```python
from build123d import *

# Parameters (mm, degrees)
F1_DEPTH = 11
F3_DEPTH = 4
F5_D     = 5


with BuildPart() as f1:
    # F0 (on Top) → F1 (new body)
    with BuildSketch(Plane.XY):
        with BuildLine():
            Line((-1.5, 17.95), (-1.5, 14.874559))
            ThreePointArc((-1.5, 14.874559), (0, -14.95), (1.5, 14.874559))
            Line((1.5, 14.874559), (1.5, 17.95))
            Line((1.5, 17.95), (-1.5, 17.95))
        make_face()
    extrude(amount=F1_DEPTH)

    # F2 (on face) → F3 (join)
    with BuildSketch(Plane.XY.offset(11)):
        with BuildLine():
            ThreePointArc((-1.5, 17.95), (-12.194951, -13.256533), (18.012565, 0))
            ThreePointArc((18.012565, 0), (13.256533, 12.194951), (1.5, 17.95))
            Line((1.5, 17.95), (1.5, 14.874559))
            ThreePointArc((1.5, 14.874559), (0, -14.95), (-1.5, 14.874559))
            Line((-1.5, 14.874559), (-1.5, 17.95))
        make_face()
        with BuildLine():
            Line((1.5, 14.874559), (1.5, 17.95))
            Line((1.5, 17.95), (-1.5, 17.95))
            Line((-1.5, 17.95), (-1.5, 14.874559))
            ThreePointArc((-1.5, 14.874559), (0, -14.95), (1.5, 14.874559))
        make_face()
    extrude(amount=F3_DEPTH)

    # F5 (through all)
    with Locations(Plane(origin=(0, 0, 0), x_dir=(1, 0, 0), z_dir=(0, 0, -1))):
        with Locations((0, 0)):
            Hole(F5_D / 2)


solid = f1.part
```
Source: CAD feature listing. Evaluate the final solid. Frame: model axes, mm. A direction names the side the tool comes from. Coordinates: 2 decimals unless noted, no trailing zeros. Write each loop counter-clockwise with the first axis right and the second up, starting at its lowest first coordinate (ties: lowest second). Pieces come first, ordered by that corner, then holes. Notation, with made-up numbers: (20, -19.75) -> (59, -19.75) arc R23 ccw to (59, 2.25) -> close; hole circle Ø1 at (10, -24). An arc over 180 degrees is marked (long way). Return JSON: item names as keys, results as strings. Group by question number.
1) Section query B-B, the plane y = -2. Return loops of the section in (x, z), plus the area to 3 significant figures.
2) Section query D-D, the plane y = 12. Return loops of the section in (x, z), plus the area to 3 significant figures.
3) Set-up query: faces 4 (the face through (1.5, 16, 5)), 5 (the face through (-1.5, 16, 5)), 6 (the face through (-4, -15, 11)). Return all of +Z, -Z, +X, -X, +Y, -Y with unobstructed straight access to the full face (end or side cutting, diameter ignored); none if empty.
4) Section query A-A, the plane x = 0. Return loops of the section in (y, z).
5) Ray query, line 1 along Y through (x, z) = (0, 5.75); line 2 along Z through (x, y) = (15, -4); line 3 along X through (y, z) = (1, 6.25). Return the intervals inside material, ascending.
6) Mould query, pull axis X, two halves, no side actions, for faces 1 (the face through (3, 2, 0)), 2 (the face through (0.54, 2.44, 7.61)), 3 (the face through (-0.636, -14.936, 5.423)). Classes: +X half, -X half, draft (parallel to the pull), parting line (faces both ways), or undercut.
7) Contact query for flat-ended pins moving along their axis: P1, Ø4, axis at y = -11, z = 2, coming from the +X side; P2, Ø6, axis at y = -1.5, z = 4.5, coming from the +X side; P3, Ø1, axis at y = 12.5, z = 7.5, coming from the +X side. Output: stop coordinate, or through.
8) Section query C-C, the plane z = 4.25. Return loops of the section in (x, y), plus the area to 3 significant figures.
From the geometry:
{
 "1": {"outline": "(-17.9, 11) -> (-14.82, 11) -> (-14.82, 0) -> (-1.5, 0) -> (-1.5, 15) -> (-17.9, 15) -> close; (1.5, 0) -> (14.82, 0) -> (14.82, 11) -> (17.9, 11) -> (17.9, 15) -> (1.5, 15) -> close", "area": "424 mm²"},
 "2": {"outline": "(-13.43, 11) -> (-8.92, 11) -> (-8.92, 0) -> (8.92, 0) -> (8.92, 11) -> (13.43, 11) -> (13.43, 15) -> (-13.43, 15) -> close", "area": "304 mm²"},
 "3": {"face 4": "-Z, +X, +Y", "face 5": "-Z, -X, +Y", "face 6": "-Z"},
 "4": {"outline": "(-18.01, 11) -> (-14.95, 11) -> (-14.95, 0) -> (-2.5, 0) -> (-2.5, 15) -> (-18.01, 15) -> close; (2.5, 0) -> (17.95, 0) -> (17.95, 15) -> (2.5, 15) -> close"},
 "5": {"line 1": "-14.95 to -2.5, 2.5 to 17.95", "line 2": "11 to 15", "line 3": "-14.92 to -2.29, 2.29 to 14.92"},
 "6": {"face 1": "draft", "face 2": "undercut", "face 3": "parting line"},
 "7": {"P1": "x = 11.94", "P2": "x = 14.95", "P3": "x = 8.92"},
 "8": {"outline": "(-1.5, 14.87) arc R14.95 ccw (long way) to (1.5, 14.87) -> (1.5, 17.95) -> (-1.5, 17.95) -> close; hole circle Ø5 at (0, 0)", "area": "692 mm²"}
}
